Work out the finished part from the listing and answer in its coordinate system (mm). Face numbers are marked on the shaded views. A direction names the side the tool comes from. Round coordinates to 2 decimals unless told otherwise and drop trailing zeros. Loops run counter-clockwise (first coordinate to the right, second up) from the corner with the lowest first, then second, coordinate; pieces in that order, holes last. Notation, with made-up numbers: (2, 79) -> (32, 79) arc R19 ccw to (32, 91) -> close; hole circle Ø8 at (-22.75, -10.75). An arc over 180 degrees is marked (long way). Use one line per item in the form item = value.
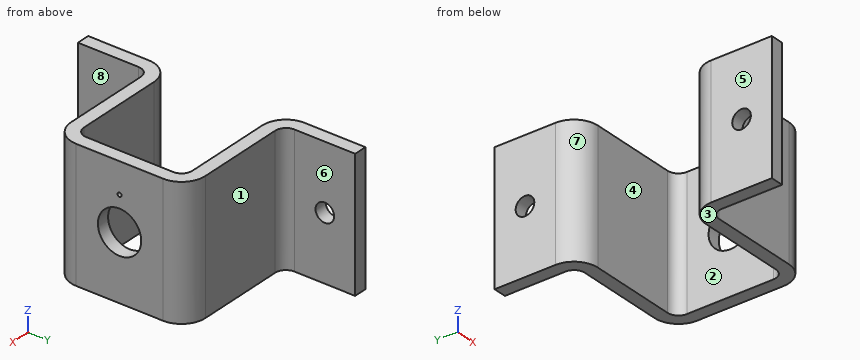
```python
from build123d import *

# Parameters (mm, degrees)
BOSS_EXTRUDE1_DEPTH       = 30
M4_CLEARANCE_HOLE1_D      = 4.3
M4_CLEARANCE_HOLE1_DEPTH  = 7
M10_CLEARANCE_HOLE1_D     = 10
M10_CLEARANCE_HOLE1_DEPTH = 7
SKETCH6_R                 = 0.475
CUT_EXTRUDE1_DEPTH        = 10


with BuildPart() as part:
    # Sketch1 → Boss-Extrude1 (new body)
    with BuildSketch(Plane.XY):
        with BuildLine():
            Line((0, 0), (0, 14))
            ThreePointArc((0, 14), (1.610912703, 17.889087297), (5.5, 19.5))
            Line((5.5, 19.5), (26, 19.5))
            ThreePointArc((26, 19.5), (27.767766953, 20.232233047), (28.5, 22))
            Line((28.5, 22), (28.5, 42))
            ThreePointArc((28.5, 42), (27.767766953, 43.767766953), (26, 44.5))
            Line((26, 44.5), (5.5, 44.5))
            ThreePointArc((5.5, 44.5), (1.610912703, 46.110912703), (0, 50))
            Line((0, 50), (0, 64))
            Line((0, 64), (3, 64))
            Line((3, 64), (3, 50))
            ThreePointArc((3, 50), (3.732233047, 48.232233047), (5.5, 47.5))
            Line((5.5, 47.5), (26, 47.5))
            ThreePointArc((26, 47.5), (29.889087297, 45.889087297), (31.5, 42))
            Line((31.5, 42), (31.5, 22))
            ThreePointArc((31.5, 22), (29.889087297, 18.110912703), (26, 16.5))
            Line((26, 16.5), (5.5, 16.5))
            ThreePointArc((5.5, 16.5), (3.732233047, 15.767766953), (3, 14))
            Line((3, 14), (3, 0))
            Line((3, 0), (0, 0))
        make_face()
    extrude(amount=BOSS_EXTRUDE1_DEPTH)

    # M4 Clearance Hole1
    with Locations(Plane(origin=(3, 0, 0), x_dir=(0, 0, -1), z_dir=(1, 0, 0))):
        with Locations((-15, 57), (-15, 7)):
            Hole(M4_CLEARANCE_HOLE1_D / 2, depth=M4_CLEARANCE_HOLE1_DEPTH)

    # M10 Clearance Hole1
    with Locations(Plane(origin=(31.5, 0, 0), x_dir=(0, 0, -1), z_dir=(1, 0, 0))):
        with Locations((-15, 32)):
            Hole(M10_CLEARANCE_HOLE1_D / 2, depth=M10_CLEARANCE_HOLE1_DEPTH)

    # Sketch6 → Cut-Extrude1 (cut)
    with BuildSketch(Plane(origin=(31.5, 0, 0), x_dir=(0, 0, -1), z_dir=(1, 0, 0))):
        with Locations((-22.92, 32)):
            Circle(SKETCH6_R)
    extrude(amount=-CUT_EXTRUDE1_DEPTH, mode=Mode.SUBTRACT)


solid = part.part
```
(1) Find section D-D, the plane z = 6.25. Write down the section's boundary in (x, y), then the cut area to 3 significant figures.
Completed:
outline = (0, 0) -> (3, 0) -> (3, 14) arc R2.5 cw to (5.5, 16.5) -> (26, 16.5) arc R5.5 ccw to (31.5, 22) -> (31.5, 42) arc R5.5 ccw to (26, 47.5) -> (5.5, 47.5) arc R2.5 cw to (3, 50) -> (3, 64) -> (0, 64) -> (0, 50) arc R5.5 ccw to (5.5, 44.5) -> (26, 44.5) arc R2.5 cw to (28.5, 42) -> (28.5, 22) arc R2.5 cw to (26, 19.5) -> (5.5, 19.5) arc R5.5 ccw to (0, 14) -> close
area = 342 mm2
(2) Find section B-B, the plane x = 10. Write down the section's boundary in (y, z), then the cut area to 3 significant figures.
Completed:
outline = (16.5, 0) -> (19.5, 0) -> (19.5, 30) -> (16.5, 30) -> close; (44.5, 0) -> (47.5, 0) -> (47.5, 30) -> (44.5, 30) -> close
area = 180 mm2
(3) Consider L1, parallel to Y at x = 12, z = 11; L2, parallel to X at y = 8.5, z = 24.25; L3, parallel to Y at x = 1.25, z = 15. Determine where each line is inside the solid, lowest interval first.
Completed:
L1 = 16.5 to 19.5, 44.5 to 47.5
L2 = 0 to 3
L3 = 0 to 4.85, 9.15 to 17.49, 46.51 to 54.85, 59.15 to 64
(4) Find section C-C, the plane y = 7. Write down the section's boundary in (x, z).
Completed:
outline = (0, 0) -> (3, 0) -> (3, 12.85) -> (0, 12.85) -> close; (0, 17.15) -> (3, 17.15) -> (3, 30) -> (0, 30) -> close
(5) Find section A-A, the plane z = 15. State how many separate pieces and enclosed holes the cut face has, then the cut area to 3 significant figures.
Completed:
separate_pieces = 4
enclosed_holes = 0
area = 287 mm2
(6) Given P1, Ø3, axis at x = 24, z = 22, coming from the +Y side; P2, Ø6, axis at x = 11.5, z = 7.5, coming from the -Y side; P3, Ø7, axis at y = 6.5, z = 20.5, coming from the +X side, each flat-ended and moving along its own axis, determine where each tip first touches the part or whether it passes through.
Completed:
P1 = 47.5
P2 = 16.5
P3 = 3
(7) For a pull along Y with two mould halves and no side action, classify the marked faces 1, 2, 3 and 4 as +Y half, -Y half, draft (parallel to the pull), parting line (faces both ways), or undercut.
Completed:
face_1 = +Y half
face_2 = undercut
face_3 = draft
face_4 = undercut
(8) For the marked faces 5, 6, 7 and 8, determine the directions among +Z, -Z, +X, -X, +Y, -Y from which every point of the face is accessible in a straight line to the end or side of a thin tool.
Completed:
face_5 = +Z, -Z, -X, +Y, -Y
face_6 = +Z, -Z, +X, +Y
face_7 = +Z, -Z, -X
face_8 = +Z, -Z, +X, -Y
